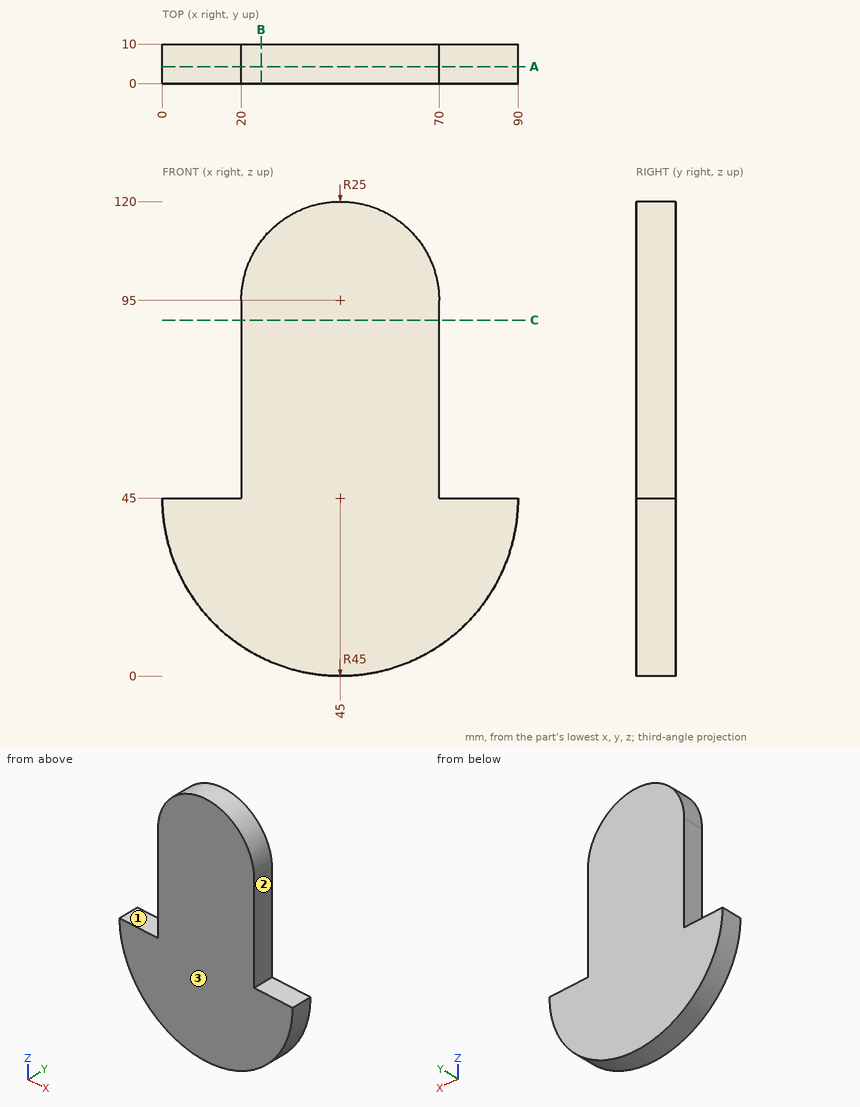
For this review, use the dimensioned drawing (mm, ordinates from the lowest corner) and the shaded views. A direction names the side the tool comes from. Give positions to 0.01 mm unless a question says otherwise; leave off trailing zeros. Loops run counter-clockwise (first coordinate to the right, second up) from the corner with the lowest first, then second, coordinate; pieces in that order, holes last. Notation, with made-up numbers: (25, -30.75) -> (53, -30.75) arc R24 cw to (53, 8.25) -> close; hole circle Ø10 at (16.5, -35). An arc over 180 degrees is marked (long way). Use CSV: the item, a comma, the result in double quotes.
1. Consider section C-C, the plane z = 90. Write out the cut boundary in (x, y).
Result:
outline,"(20, 0) -> (70, 0) -> (70, 10) -> (20, 10) -> close"
2. Consider section B-B, the plane x = 25. Write out the cut boundary in (y, z).
Result:
outline,"(0, 4.69) -> (10, 4.69) -> (10, 110) -> (0, 110) -> close"
3. To check wall thickness, follow probe 1 along X at (y, z) = (5, 50.5); probe 2 along Z at (x, y) = (54.5, 4.25); probe 3 along Z at (x, y) = (86.5, 4.75). State the ranges of each line that lie inside material, in increasing order. Write a range as from..to.
Result:
probe 1,"x = 20..70"
probe 2,"z = 1.01..118.12"
probe 3,"z = 27.6..45"
4. Consider section A-A, the plane y = 4.25. Write out the cut boundary in (x, z), then the cut area to 3 significant figures.
Result:
outline,"(0, 45) arc R45 ccw to (90, 45) -> (70, 45) -> (70, 95) arc R25 ccw to (20, 95) -> (20, 45) -> close"
area,"6,660 mm²"
5. For P1, Ø2, axis at y = 9, z = 67, coming from the -X side; P2, Ø3, axis at y = 5.5, z = 98.5, coming from the -X side; P3, Ø4, axis at x = 51.5, y = 4, coming from the -Z side, all flat-tipped, find the tip position at first contact; note any pin that passes through.
Result:
P1,"stops at x = 20"
P2,"stops at x = 20.08"
P3,"stops at z = 0.23"
6. Machinability: for the marked faces 1, 2 and 3, which of the approach directions +Z, -Z, +X, -X, +Y, -Y give a long, thin tool a straight path to every point of the face, cutting with its end or side? Answer none if there is none.
Result:
face 1,"+Z, -X, +Y, -Y"
face 2,"+Z, +X, +Y, -Y"
face 3,"+Z, -Z, +X, -X, -Y"
